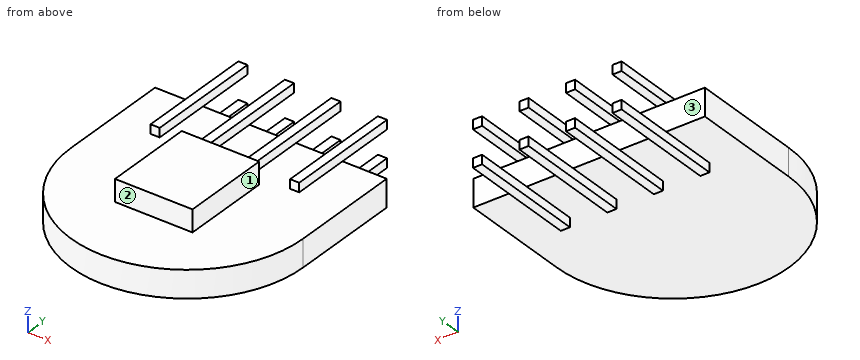
```python
from build123d import *

# Parameters (mm, degrees)
P_IDAT_VYSUNUT_M1_DEPTH  = 1.5
P_IDAT_START             = 1.5
SKICA1_3_W               = 4.25
SKICA1_3_H               = 4.94
P_IDAT_VYSUNUT_M2_DEPTH  = 1.2
SKICA3_W                 = 12.7
SKICA3_H                 = 1.5
ODEBRAT_VYSUNUT_M1_DEPTH = 3.5
SKICA4_W                 = 12.7
SKICA4_H                 = 1.5
ODEBRAT_VYSUNUT_M2_DEPTH = 5.5
SKICA7_W                 = 12.7
SKICA7_H                 = 1.5
P_IDAT_VYSUNUT_M5_DEPTH  = 2.7055
P_IDAT_START_2           = 3
SKICA15_W                = 0.5
SKICA15_H                = 0.5
P_IDAT_VYSUNUT_M14_DEPTH = 6.5
LINPOLE3_COUNT           = 4
LINPOLE3_PITCH           = 2.55
LINPOLE4_COUNT           = 2
LINPOLE4_PITCH           = 2
LINPOLE4_START           = 3
LINPOLE4_COPY_1_SKETCH_W = 0.5
LINPOLE4_COPY_1_SKETCH_H = 0.5
LINPOLE4_COPY_1_DEPTH    = 6.5
LINPOLE4_COPY_2_SKETCH_W = 0.5
LINPOLE4_COPY_2_SKETCH_H = 0.5
LINPOLE4_COPY_2_DEPTH    = 6.5
LINPOLE4_COPY_3_SKETCH_W = 0.5
LINPOLE4_COPY_3_SKETCH_H = 0.5
LINPOLE4_COPY_3_DEPTH    = 6.5


with BuildPart() as part:
    # Skica1 → Přidat vysunutím1 (new body)
    with BuildSketch(Plane.XY):
        with BuildLine():
            Line((-6.35, 0), (-6.35, 12.5))
            Line((-6.35, 12.5), (6.35, 12.5))
            Line((6.35, 12.5), (6.35, 0))
            ThreePointArc((6.35, 0), (0, -6.35), (-6.35, 0))
        make_face()
    extrude(amount=P_IDAT_VYSUNUT_M1_DEPTH)

    # Skica1<3> → Přidat vysunutím2 (add)
    with BuildSketch(Plane.XY.offset(P_IDAT_START)):
        Rectangle(SKICA1_3_W, SKICA1_3_H)
    extrude(amount=P_IDAT_VYSUNUT_M2_DEPTH)

    # Skica3 → Odebrat vysunutím1 (cut)
    with BuildSketch(Plane(origin=(0, 12.5, 0), x_dir=(1, 0, 0), z_dir=(0, 1, 0))):
        with Locations((0, -0.75)):
            Rectangle(SKICA3_W, SKICA3_H)
    extrude(amount=-ODEBRAT_VYSUNUT_M1_DEPTH, mode=Mode.SUBTRACT)

    # Skica4 → Odebrat vysunutím2 (cut)
    with BuildSketch(Plane(origin=(0, 9, 0), x_dir=(1, 0, 0), z_dir=(0, 1, 0))):
        with Locations((0, -0.75)):
            Rectangle(SKICA4_W, SKICA4_H)
    extrude(amount=-ODEBRAT_VYSUNUT_M2_DEPTH, mode=Mode.SUBTRACT)

    # Skica7 → Přidat vysunutím5 (add)
    with BuildSketch(Plane(origin=(0, 3.5, 0), x_dir=(1, 0, 0), z_dir=(0, 1, 0))):
        with Locations((0, -0.75)):
            Rectangle(SKICA7_W, SKICA7_H)
    extrude(amount=P_IDAT_VYSUNUT_M5_DEPTH)

    # Skica15 → Přidat vysunutím14 (add)
    with BuildSketch(Plane(origin=(0, 0, 0), x_dir=(1, 0, 0), z_dir=(0, 1, 0)).offset(P_IDAT_START_2)):
        with Locations((-3.975, -1.75)):
            Rectangle(SKICA15_W, SKICA15_H)
    p_idat_vysunut_m14 = extrude(amount=P_IDAT_VYSUNUT_M14_DEPTH)

    # LinPole3: Přidat vysunutím14 ×4
    with Locations(*[(i * LINPOLE3_PITCH, 0, 0) for i in range(1, LINPOLE3_COUNT)]):
        add(p_idat_vysunut_m14)

    # LinPole4: Přidat vysunutím14 ×2
    with Locations(*[(0, 0, -i * LINPOLE4_PITCH) for i in range(1, LINPOLE4_COUNT)]):
        add(p_idat_vysunut_m14)

    # LinPole4 copy 1 sketch → LinPole4 copy 1 (add)
    with BuildSketch(Plane(origin=(2.55, 0, -2), x_dir=(1, 0, 0), z_dir=(0, 1, 0)).offset(LINPOLE4_START)):
        with Locations((-3.975, -1.75)):
            Rectangle(LINPOLE4_COPY_1_SKETCH_W, LINPOLE4_COPY_1_SKETCH_H)
    extrude(amount=LINPOLE4_COPY_1_DEPTH)

    # LinPole4 copy 2 sketch → LinPole4 copy 2 (add)
    with BuildSketch(Plane(origin=(5.1, 0, -2), x_dir=(1, 0, 0), z_dir=(0, 1, 0)).offset(LINPOLE4_START)):
        with Locations((-3.975, -1.75)):
            Rectangle(LINPOLE4_COPY_2_SKETCH_W, LINPOLE4_COPY_2_SKETCH_H)
    extrude(amount=LINPOLE4_COPY_2_DEPTH)

    # LinPole4 copy 3 sketch → LinPole4 copy 3 (add)
    with BuildSketch(Plane(origin=(7.65, 0, -2), x_dir=(1, 0, 0), z_dir=(0, 1, 0)).offset(LINPOLE4_START)):
        with Locations((-3.975, -1.75)):
            Rectangle(LINPOLE4_COPY_3_SKETCH_W, LINPOLE4_COPY_3_SKETCH_H)
    extrude(amount=LINPOLE4_COPY_3_DEPTH)


solid = part.part
```
For this review, take the finished solid that the model builds, in its own axes (mm). Face numbers are marked on the shaded views. A direction names the side the tool comes from. Give positions to 0.01 mm unless a question says otherwise; leave off trailing zeros. Write each loop counter-clockwise with the first axis right and the second up, starting at its lowest first coordinate (ties: lowest second). Pieces come first, ordered by that corner, then holes. Notation, with made-up numbers: M -20,16.5 L -4,16.5 A3 cw -4,20.5 Z; hole C -21,70.5 d7. An arc over 180 degrees is marked long. One line per item, written item: value.
1) Take a section at D-D, the plane z = 1. Write out the cut boundary in (x, y).
Results are:
outline: M -6.35,0 A6.35 ccw 6.35,0 L 6.35,6.21 L -6.35,6.21 Z
2) Take a section at A-A, the plane y = 8.75. Count the separate pieces of the cut face and the enclosed holes in it, then the cut area to 3 significant figures.
Results are:
separate pieces: 8
enclosed holes: 0
area: 2.00 mm²
3) Take a section at C-C, the plane x = 0. Write out the cut boundary in (y, z), then the cut area to 3 significant figures.
Results are:
outline: M -6.35,0 L 6.21,0 L 6.21,1.5 L 2.47,1.5 L 2.47,2.7 L -2.47,2.7 L -2.47,1.5 L -6.35,1.5 Z
area: 24.8 mm²
4) For the marked faces 1, 2 and 3, list the 3-axis set-ups (+Z, -Z, +X, -X, +Y, -Y) from which the entire face can be reached by the end or side of a thin tool; tool diameter is ignored.
Results are:
face 1: +Z, +X, +Y, -Y
face 2: +Z, +X, -X, -Y
face 3: +X, -X, +Y
5) Take a section at B-B, the plane y = 0.25. Write out the cut boundary in (x, z) (3 decimals), then the cut area to 4 significant figures.
Results are:
outline: M -6.35,0 L 6.35,0 L 6.35,1.5 L 2.125,1.5 L 2.125,2.7 L -2.125,2.7 L -2.125,1.5 L -6.35,1.5 Z
area: 24.15 mm²
6) For P1, Ø0.8, axis at x = -1, z = 0.5, coming from the +Y side; P2, Ø1, axis at y = -2, z = 0.5, coming from the -X side; P3, Ø0.6, axis at y = 7.5, z = -0.5, coming from the -X side (3 decimals), all flat-tipped, find the tip position at first contact; note any pin that passes through.
Results are:
P1: stops at y = 6.21
P2: stops at x = -6.17
P3: stops at x = -4.225
7) For line 1 (X direction, y = 3.25, z = 1.9) (3 decimals); line 2 (Z direction, x = -4.75, y = -1.75); line 3 (Z direction, x = 3.75, y = 5.75), list the stretches that pass through material, from the lowest coordinate up. Write a range as from..to.
Results are:
line 1: x = -4.225..-3.725, -1.675..-1.175, 0.875..1.375, 3.425..3.925
line 2: z = 0..1.5
line 3: z = -0.5..2
